For this review, take the finished solid that the model builds, in its own axes (mm). Face numbers are marked on the shaded views. A direction names the side the tool comes from. Round coordinates to 2 decimals unless told otherwise and drop trailing zeros. Order: outer loops, then holes, each group sorted by start corner. A loop starts at its lowest first (then second) coordinate and runs counter-clockwise, first axis right, second up. Notation, with made-up numbers: M 87,18.5 L 91,18.5 A17 cw 91,33.5 Z; hole C 22.25,-21.75 d10. An arc over 180 degrees is marked long. Answer as a JSON object with one key per item and string values.
from build123d import *

# Parameters (mm, degrees)
SKETCH1_R             = 25
BOTTOM_CYLINDER_DEPTH = 20
SKETCH3_R             = 15
SKETCH2_R             = 25
SKETCH5_R             = 1.5
UVC_RODS_DEPTH        = 80
SKETCH6_R             = 25
TOP_DEPTH             = 10
FILLET1_R             = 10
LIDAR_CUBBY_REACH     = 98.695
SKETCH8_W             = 6
SKETCH8_H             = 6
BOSS_EXTRUDE1_REACH   = 80.422
SKETCH9_R             = 5


with BuildPart() as part:
    # Sketch1 → Bottom-cylinder (new body)
    with BuildSketch(Plane(origin=(0, 0, 0), x_dir=(1, 0, 0), z_dir=(0, 1, 0))):
        with Locations(Location((0, 0, 0), (0, 0, 270))):
            Circle(SKETCH1_R)
    extrude(amount=BOTTOM_CYLINDER_DEPTH)

    # Sketch3 → Cone-top section 0
    with BuildSketch(Plane(origin=(0, 40, 0), x_dir=(-1, 0, 0), z_dir=(0, -1, 0))):
        Circle(SKETCH3_R)
    # Sketch2 → Cone-top section 1
    with BuildSketch(Plane(origin=(0, 20, 0), x_dir=(1, 0, 0), z_dir=(0, 1, 0))):
        Circle(SKETCH2_R)
    loft()

    # Sketch5 → UVC-rods (add)
    with BuildSketch(Plane(origin=(0, 20, 0), x_dir=(1, 0, 0), z_dir=(0, 1, 0))):
        with Locations(Location((0, 20, 0), (0, 0, 90.000009577))):
            Circle(SKETCH5_R)
        with Locations(Location((17.320508076, -10, 0), (0, 0, 0.247467178))):
            Circle(SKETCH5_R)
        with Locations(Location((-17.320508076, -10, 0), (0, 0, 183.11947614))):
            Circle(SKETCH5_R)
    extrude(amount=UVC_RODS_DEPTH)

    # Sketch6 → Top (add)
    with BuildSketch(Plane(origin=(0, 100, 0), x_dir=(1, 0, 0), z_dir=(0, 1, 0))):
        with Locations(Location((0, 0, 0), (0, 0, 90))):
            Circle(SKETCH6_R)
    extrude(amount=TOP_DEPTH)

    # Fillet1
    fillet1_edges = [part.edges().sort_by_distance(p)[0] for p in [
        (0, 110, 25),
    ]]
    fillet(fillet1_edges, radius=FILLET1_R - 0.0001)  # a hair under: the kernel refuses the full size

    # Lidar-cubby: up to this cone (the profile starts inside it)
    lidar_cubby_end = Plane(origin=(0, 20, 0), z_dir=(0, -1, 0)).offset(-49.999999) * Cone(1e-06, 87.0975, 174.194999, align=(Align.CENTER, Align.CENTER, Align.MIN), mode=Mode.PRIVATE)
    # Sketch8 → Lidar-cubby (cut, up to the surface)
    with BuildSketch(Plane(origin=(0, 20, 0), x_dir=(1, 0, 0), z_dir=(0, 1, 0)), mode=Mode.PRIVATE) as lidar_cubby_sk1:
        with Locations((0, -22)):
            Rectangle(SKETCH8_W, SKETCH8_H)
    lidar_cubby_tool1 = extrude(lidar_cubby_sk1.sketch, amount=LIDAR_CUBBY_REACH, mode=Mode.PRIVATE) & lidar_cubby_end
    add(lidar_cubby_tool1.solids().sort_by_distance((0, 20, 22))[0], mode=Mode.SUBTRACT)

    # Sketch9 → Boss-Extrude1 (add, up to next)
    with BuildSketch(Plane(origin=(0, 40, 0), x_dir=(1, 0, 0), z_dir=(0, 1, 0)), mode=Mode.PRIVATE) as boss_extrude1_sk1:
        with Locations(Location((0, 0, 0), (0, 0, 270))):
            Circle(SKETCH9_R)
    boss_extrude1_tool1 = extrude(boss_extrude1_sk1.sketch, amount=BOSS_EXTRUDE1_REACH, mode=Mode.PRIVATE) - part.part
    add(boss_extrude1_tool1.solids().sort_by_distance((0, 40, 0))[0])


solid = part.part
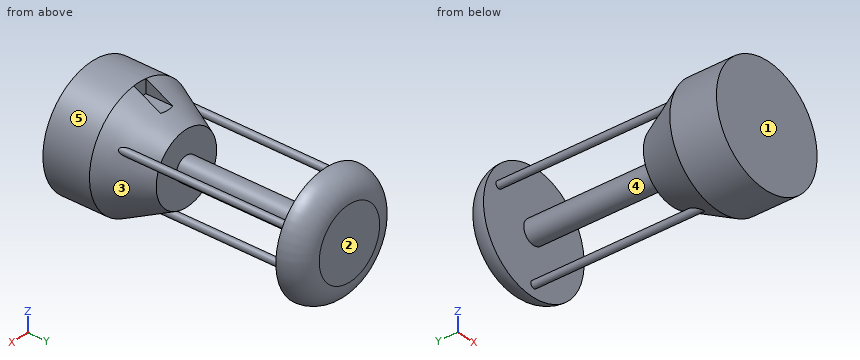
1) Add section B-B on y = 38. State the section outline as (x, z) points, and give its area (3 significant figures).
Geometry check:
{"outline": "C -17.32,10 d3; C 0,0 d32; C 0,-20 d3; C 17.32,10 d3", "area": "825 mm²"}
2) Machinability: for the marked faces 4 and 5, which of the approach directions +Z, -Z, +X, -X, +Y, -Y give a long, thin tool a straight path to every point of the face, cutting with its end or side? Answer none if there is none.
Geometry check:
{"face 4": "none", "face 5": "+Y, -Y"}
3) Add section C-C on y = 17.5. State the section outline as (x, z) points.
Geometry check:
{"outline": "C 0,0 d50"}
4) For L1, parallel to Y at x = 10, z = -2; L2, parallel to Y at x = -8, z = -20.5; L3, parallel to X at y = 88.5, z = 4, list the stretches that pass through material, from the lowest coordinate up.
Geometry check:
{"L1": "y = 0 to 40, 100 to 110", "L2": "y = 0 to 25.99, 100 to 107.14", "L3": "x = -3 to 3"}
5) Insertion check: P1, Ø1.7, axis at y = 23, z = 20.5, coming from the -X side; P2, Ø6, axis at y = 92, z = -17.5, coming from the +X side; P3, Ø6.5, axis at x = 0, y = 25.5, coming from the +Z side. Each pin has a flat end and moves straight along its axis. Give the tip position at first contact, or say it passes through.
Geometry check:
{"P1": "stops at x = -13.1", "P2": "stops at x = 1.5", "P3": "stops at z = 22.68"}
6) Mouldability with a two-part tool opening along Y and no side actions: class the marked faces 1, 2 and 3 as +Y half, -Y half, draft (parallel to the pull), parting line (faces both ways), or undercut.
Geometry check:
{"face 1": "-Y half", "face 2": "+Y half", "face 3": "undercut"}
